Input: part model. Units: mm. Frame: model coordinates. Coordinates: 2 decimals unless noted, no trailing zeros. Loops run counter-clockwise (first coordinate to the right, second up) from the corner with the lowest first, then second, coordinate; pieces in that order, holes last. Notation, with made-up numbers: (2, 7) - (40, 7) arc R23 ccw to (40, 20) - close; hole circle Ø4 at (31, -28). An arc over 180 degrees is marked (long way). Use one line per item in the form item = value.
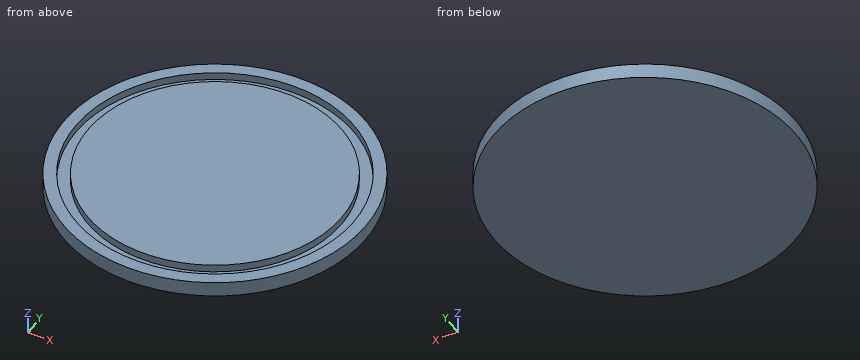
from build123d import *

# Parameters (mm, degrees)
F0_R     = 25
F0_R_2   = 23
F0_R_3   = 21
F1_DEPTH = 1.25
F2_DEPTH = 25


with BuildPart() as f1:
    # F0 (on Top) → F1 (new body, symmetric)
    with BuildSketch(Plane.XY):
        Circle(F0_R)
        Circle(F0_R_2, mode=Mode.SUBTRACT)
        Circle(F0_R_2)
        Circle(F0_R_3, mode=Mode.SUBTRACT)
        Circle(F0_R_3)
    extrude(amount=F1_DEPTH, both=True)

    # F0 (on Top) → F2 (cut)
    with BuildSketch(Plane.XY):
        Circle(F0_R_2)
        Circle(F0_R_3, mode=Mode.SUBTRACT)
    extrude(amount=F2_DEPTH, mode=Mode.SUBTRACT)


solid = f1.part
Q1. Cut plane A-A, the plane z = 0.5. Return loops of the section in (x, y), then the cut area to 3 significant figures.
Check values:
outline = circle Ø50 at (0, 0); circle Ø42 at (0, 0); hole circle Ø46 at (0, 0)
area = 1,690 mm²
Q2. Ray query, line 1 along Y through (x, z) = (0, 0.5); line 2 along Y through (x, z) = (-11, 0.1); line 3 along X through (y, z) = (-19.5, -0.8). Return the intervals inside material, ascending. Write a range as [from, to].
Check values:
line_1 = [-25, -23], [-21, 21], [23, 25]
line_2 = [-22.45, -20.2], [-17.89, 17.89], [20.2, 22.45]
line_3 = [-15.64, 15.64]
Q3. Cut plane B-B, the plane x = 0. Return loops of the section in (y, z), then the cut area to 3 significant figures.
Check values:
outline = (-25, -1.25) - (25, -1.25) - (25, 1.25) - (23, 1.25) - (23, 0) - (21, 0) - (21, 1.25) - (-21, 1.25) - (-21, 0) - (-23, 0) - (-23, 1.25) - (-25, 1.25) - close
area = 120 mm²
